Autodesk Inventor part; units mm, degrees
ref_plane "YZ Plane" through (0, 0, 0) normal (1, 0, 0) x (0, 1, 0)
ref_plane "XZ Plane" through (0, 0, 0) normal (0, 1, 0) x (-1, 0, 0)
ref_plane "XY Plane" through (0, 0, 0) normal (0, 0, 1) x (1, 0, 0)
sketch "Эскиз1" plane through (0, 0, 0) normal (0, 1, 0) x (-1, 0, 0)
  circle A0 centre (0, 0) radius 50
  circle A1 centre (0, 40) radius 40
  line L0 (44.1832, 40) -> (-44.0888, 40)
  line L1 (0.3076, 84.5902) -> (0.3076, -55.7597)
  line L2 (55.3799, 0) -> (-56.0667, 0)
  dimension "d0" = 100
  dimension "d2" = 80
sketch "Эскиз2" plane through (0, 0, 0) normal (1, 0, 0) x (0, 1, 0)
  line L0 (0, 40.0046) -> (100, 40.0046)
  line L1 (0, 40.0046) -> (0, 80.0046)
  line L2 (0, 80.0046) -> (100, 40.0046)
  line L3 (0, 0) -> (80, 0)
  line L4 (0, 0) -> (0, -50)
  line L5 (0, -50) -> (80, 0)
  dimension "d3" = 100
  dimension "d4" = 40
  dimension "d5" = 80
  dimension "d6" = 50
revolve "Вращение1" add sketch "Эскиз2" angle 360 about axis through (0, 0, 40.0046) along (0, 1, 0) contours L1 L2 L0
revolve "Вращение2" add sketch "Эскиз2" angle 360 about axis through (0, 0, 0) along (0, 1, 0) contours L3 L5 L4
ref_plane "РабПлоскость1" through (0, 33.25, 0) normal (0, -1, 0) x (1, 0, 0)
split_face "Разделение1"
split_face "Разделение2"
ref_plane "РабПлоскость2" through (0, 100, 0) normal (0, -1, 0) x (1, 0, 0)
ref_plane "РабПлоскость3" through (0, 80, 0) normal (0, -1, 0) x (1, 0, 0)
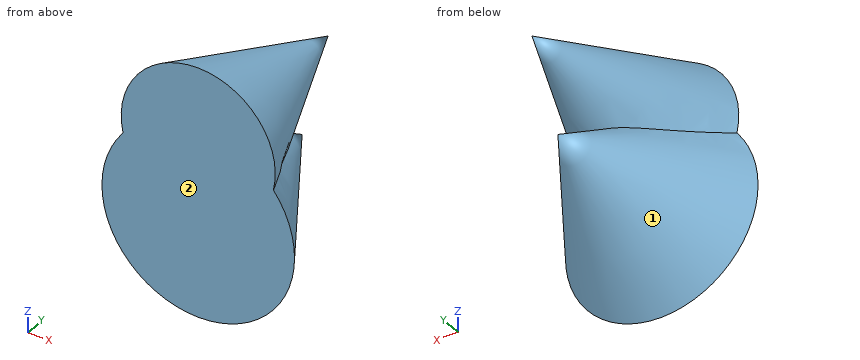
Input: part model. Units: mm. Frame: model coordinates. Face numbers are marked on the shaded views. Coordinates: 2 decimals unless noted, no trailing zeros. Write each loop counter-clockwise with the first axis right and the second up, starting at its lowest first coordinate (ties: lowest second). Pieces come first, ordered by that corner, then holes.
1) Section C-C on y = 68.5. Output: boundary loops of the cut face in (x, z) (1 decimal).
2) Mould query, pull axis Z, two halves, no side actions, for the marked faces 1 and 2. Classes: pulls with the +Z half, pulls with the -Z half, needs draft (parallel to the pull), parting line crosses it, or undercut.
3) Pin query (flat end, axial travel): pin 1 Ø3 at (y, z) = (26, 50) entering from -X; pin 2 Ø8 at (y, z) = (26.5, -9) entering from -X; pin 3 Ø1 at (y, z) = (30.5, 6) entering from -X. Return the tip coordinate at first contact, or that it passes through.
4) Material intervals for line 1 along X through (y, z) = (45.5, 44); line 2 along Y through (x, z) = (-24, 0.5); line 3 along Y through (x, z) = (-28.5, -8.5), sorted ascending.
5) Section D-D on y = 35. Output: boundary loops of the cut face in (x, z) (3 decimals).
6) Section B-B on y = 14.5. Output: boundary loops of the cut face in (x, z) (1 decimal).
7) Section A-A on y = 50. Output: boundary loops of the cut face in (x, z).
Check result:
1. outline: circle Ø25.2 at (0, 40); circle Ø14.4 at (0, 0)
2. face 1: undercut
2. face 2: needs draft
3. pin 1: stops at x = -28.67
3. pin 2: stops at x = -34.96
3. pin 3: stops at x = -30.68
4. line 1: x = -21.43 to 21.43
4. line 2: y = 0 to 41.59
4. line 3: y = 0 to 32.42
5. outline: (-18.203, 21.44) arc R28.125 ccw (long way) to (18.203, 21.44) arc R26 ccw (long way) to start
6. outline: (-31.3, 26.3) arc R40.9 ccw (long way) to (31.3, 26.3) arc R34.2 ccw (long way) to start
7. outline: circle Ø40 at (0, 40); circle Ø37.5 at (0, 0)
